Here's the drawing with two shaded views (mm, measured from the low corner). I have some questions. Give positions to 0.01 mm unless a question says otherwise; leave off trailing zeros. Loops run counter-clockwise (first coordinate to the right, second up) from the corner with the lowest first, then second, coordinate; pieces in that order, holes last. Notation, with made-up numbers: (74.25, 37.5) - (129.25, 37.5) arc R26 ccw to (129.25, 51.5) - close; hole circle Ø11 at (-38, -37.5). An arc over 180 degrees is marked (long way). Answer as a JSON object with one key per item and string values. Group by question number.
Item 1: Please list where these lines run through material, in increasing order: L1, parallel to Y at x = 13.9, z = 0.4; L2, parallel to Y at x = 9.5, z = 0.65; L3, parallel to X at y = 6, z = 0.35.
Item 2: Suppose I cut it at A-A on y = 12. Write out the boundary of the cut face in (x, z).
Item 3: Suppose I cut it at D-D on x = 5. Write out the boundary of the cut face in (y, z), and give its area (3 significant figures).
Item 4: Suppose I cut it at C-C on z = 0.65. Write out the boundary of the cut face in (x, y).
Item 5: Will these pins go through, and if not, where does the flat tip stop? pin 1 (0.5 mm diameter, centred on y = 15, z = 0.5, fed in from +X); pin 2 (1 mm diameter, centred on x = 12, y = 34.5, fed in from -Z); pin 3 (0.5 mm diameter, centred on y = 22, z = 0.5, fed in from -X); pin 4 (0.5 mm diameter, centred on x = 27, z = 0.5, fed in from -Y).
Item 6: Suppose I cut it at B-B on x = 13.9. Write out the boundary of the cut face in (y, z), and give its area (3 significant figures).
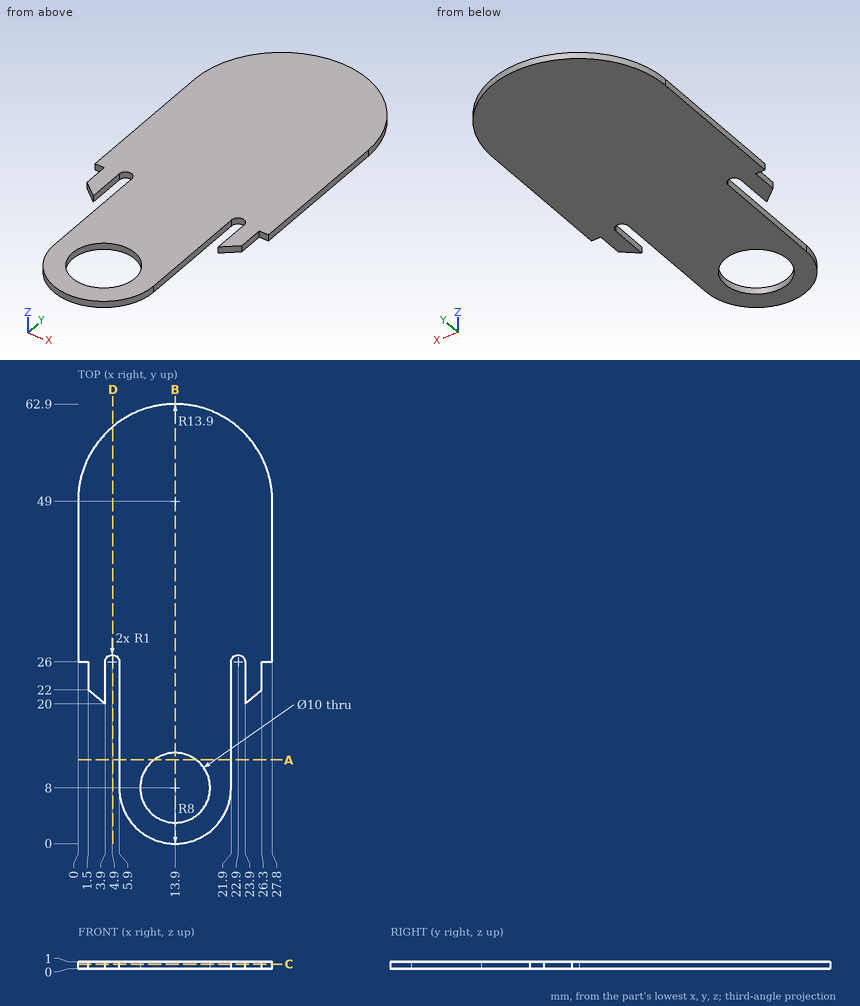
Worked out:
{
 "1": {"L1": "y = 0 to 3, 13 to 62.9", "L2": "y = 1.32 to 5.63, 10.37 to 62.19", "L3": "x = 6.15 to 9.32, 18.48 to 21.65"},
 "2": {"outline": "(5.9, 0) - (10.9, 0) - (10.9, 1) - (5.9, 1) - close; (16.9, 0) - (21.9, 0) - (21.9, 1) - (16.9, 1) - close"},
 "3": {"outline": "(26.99, 0) - (59.68, 0) - (59.68, 1) - (26.99, 1) - close", "area": "32.7 mm2"},
 "4": {"outline": "(0, 26) - (1.5, 26) - (1.5, 22) - (3.9, 20) - (3.9, 26) arc R1 cw to (5.9, 26) - (5.9, 8) arc R8 ccw to (21.9, 8) - (21.9, 26) arc R1 cw to (23.9, 26) - (23.9, 20) - (26.3, 22) - (26.3, 26) - (27.8, 26) - (27.8, 49) arc R13.9 ccw to (0, 49) - close; hole circle Ø10 at (13.9, 8)"},
 "5": {"pin 1": "stops at x = 21.9", "pin 2": "stops at z = 0", "pin 3": "stops at x = 1.5", "pin 4": "stops at y = 26"},
 "6": {"outline": "(0, 0) - (3, 0) - (3, 1) - (0, 1) - close; (13, 0) - (62.9, 0) - (62.9, 1) - (13, 1) - close", "area": "52.9 mm2"}
}
